```python
from build123d import *

# Parameters (mm, degrees)
F0_W          = 30
F0_H          = 50
F1_DEPTH      = 60
F0_W_2        = 70
F2_DEPTH      = 20
F4_DEPTH      = 71.1
F6_DEPTH      = 5
F6_DEPTH_BACK = 5
F8_DEPTH      = 205.9


with BuildPart() as f1:
    # F0 (on Top) → F1 (new body)
    with BuildSketch(Plane.XY):
        with Locations((-35, 0)):
            Rectangle(F0_W, F0_H)
    extrude(amount=F1_DEPTH)

    # F0 (on Top) → F2 (join)
    with BuildSketch(Plane.XY):
        with Locations((15, 0)):
            Rectangle(F0_W_2, F0_H)
    extrude(amount=F2_DEPTH)

    # F3 (on face) → F4 (cut)
    with BuildSketch(Plane.XY.offset(60)):
        with BuildLine():
            ThreePointArc((-50, -15), (-39.3933982822, -10.6066017178), (-35, 0))
            ThreePointArc((-35, 0), (-39.3933982822, 10.6066017178), (-50, 15))
            Line((-50, 15), (-50, -15))
        make_face()
    extrude(amount=-F4_DEPTH, mode=Mode.SUBTRACT)

    # F5 (on Front) → F6 (join, two sides)
    with BuildSketch(Plane.XZ) as f6_sk:
        Polygon((-20, 20), (50, 20), (-20, 60), align=None)
    extrude(amount=F6_DEPTH)
    extrude(f6_sk.sketch, amount=-F6_DEPTH_BACK)

    # F7 (on face) → F8 (cut)
    with BuildSketch(Plane.XZ.offset(25)):
        Polygon((0, 0), (30, 0), (40, 10), (-10, 10), align=None)
    extrude(amount=-F8_DEPTH, mode=Mode.SUBTRACT)


solid = f1.part
```
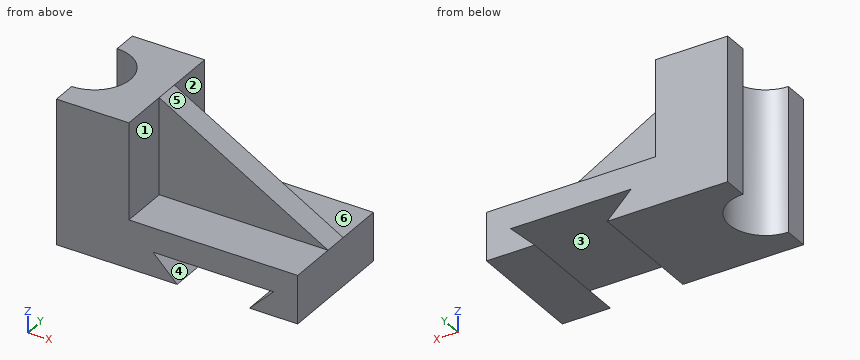
Design review of the part built by this model. Coordinates are the model's own, in mm. Face numbers are marked on the shaded views. A direction names the side the tool comes from. Coordinates: 2 decimals unless noted, no trailing zeros. Order: outer loops, then holes, each group sorted by start corner. A loop starts at its lowest first (then second) coordinate and runs counter-clockwise, first axis right, second up. Notation, with made-up numbers: (15, -9.75) - (72, -9.75) arc R6 cw to (72, -1.75) - close; hole circle Ø10 at (29, 54.25). An arc over 180 degrees is marked (long way). One line per question, with ' | ' between items.
Q1. The part is to be moulded in two halves that separate along X. For the marked faces 4, 5 and 6, say which applies: +X half, -X half, draft (parallel to the pull), parting line (faces both ways), or undercut.
Answer key:
face 4: undercut | face 5: +X half | face 6: draft
Q2. Consider section C-C, the plane x = -5.5. Give the boundary of the cut face in (y, z).
Answer key:
outline: (-25, 0) - (25, 0) - (25, 5.5) - (-25, 5.5) - close; (-25, 10) - (25, 10) - (25, 20) - (5, 20) - (5, 51.71) - (-5, 51.71) - (-5, 20) - (-25, 20) - close
Q3. Clearance check with flat-ended pins moving along their axes: pin 1 Ø20 at (x, z) = (6, 40) entering from +Y; pin 2 Ø10 at (x, y) = (16, 14.5) entering from +Z; pin 3 Ø10 at (y, z) = (-11, 31.5) entering from +X; pin 4 Ø3 at (x, z) = (12.5, 44.5) entering from +Y. State where each tip first meets the part, or that it passes through.
Answer key:
pin 1: stops at y = 5 | pin 2: stops at z = 20 | pin 3: stops at x = -20 | pin 4: passes through
Q4. Consider section D-D, the plane z = 47. Give the boundary of the cut face in (x, y).
Answer key:
outline: (-50, -25) - (-20, -25) - (-20, -5) - (2.75, -5) - (2.75, 5) - (-20, 5) - (-20, 25) - (-50, 25) - (-50, 15) arc R15 cw to (-50, -15) - close
Q5. Consider section B-B, the plane y = 0. Give the boundary of the cut face in (x, z).
Answer key:
outline: (-35, 0) - (0, 0) - (-10, 10) - (40, 10) - (30, 0) - (50, 0) - (50, 20) - (-20, 60) - (-35, 60) - close
Q6. To check wall thickness, follow line 1 along Y through (x, z) = (-1.5, 42); line 2 along Y through (x, z) = (-41, 5); line 3 along Z through (x, y) = (36, 12). State the ranges of each line that lie inside material, in increasing order.
Answer key:
line 1: y = -5 to 5 | line 2: y = -25 to -12, 12 to 25 | line 3: z = 0 to 6, 10 to 20
Q7. Consider section A-A, the plane z = 7. Give the boundary of the cut face in (x, y), then the cut area to 3 significant figures.
Answer key:
outline: (-50, -25) - (-7, -25) - (-7, 25) - (-50, 25) - (-50, 15) arc R15 cw to (-50, -15) - close; (37, -25) - (50, -25) - (50, 25) - (37, 25) - close | area: 2,450 mm2
Q8. For the marked faces 1, 2 and 3, list the 3-axis set-ups (+Z, -Z, +X, -X, +Y, -Y) from which the entire face can be reached by the end or side of a thin tool; tool diameter is ignored.
Answer key:
face 1: +Z, +X, -Y | face 2: +Z, +X, +Y | face 3: +Y, -Y
